from build123d import *

# Parameters (mm, degrees)
F0_W     = 120
F0_H     = 120
F1_DEPTH = 60
F2_W     = 100
F2_H     = 100
F3_DEPTH = 50
F4_R     = 10
F5_R     = 9
F6_DEPTH = 5
F7_R     = 10
F9_DEPTH = 45


with BuildPart() as f1:
    # F0 (on Top) → F1 (new body)
    with BuildSketch(Plane.XY):
        with Locations((-63.325952, -55.072633)):
            Rectangle(F0_W, F0_H)
    extrude(amount=F1_DEPTH)

    # F2 (on face) → F3 (cut)
    with BuildSketch(Plane.XY.offset(60)):
        with Locations((-53.325952, -65.072633)):
            Rectangle(F2_W, F2_H)
    extrude(amount=-F3_DEPTH, mode=Mode.SUBTRACT)

    # F4
    f4_edges = [f1.edges().sort_by_distance(p)[0] for p in [
        (-103.325952, -15.072633, 35),
        (-53.325952, -15.072633, 10),
        (-103.325952, -65.072633, 10),
    ]]
    fillet(f4_edges, radius=F4_R)

    # F5 (on face) → F6 (cut)
    with BuildSketch(Plane.XY.offset(60)):
        with Locations((-63.533046, -10.001782)):
            Circle(F5_R)
    extrude(amount=-F6_DEPTH, mode=Mode.SUBTRACT)

    # F7
    f7_edges = [f1.edges().sort_by_distance(p)[0] for p in [
        (-123.325952, 4.927367, 30),
    ]]
    fillet(f7_edges, radius=F7_R)

    # F8 (on face) → F9 (join)
    with BuildSketch(Plane.XY.offset(10)):
        with BuildLine():
            ThreePointArc((-63.325952, -1.072633), (-72.325952, -10.072633), (-63.325952, -19.072633))
            Line((-63.325952, -19.072633), (-63.325952, -1.072633))
        make_face()
        with BuildLine():
            Line((-63.325952, -1.072633), (-63.325952, -19.072633))
            ThreePointArc((-63.325952, -19.072633), (-56.96199, -16.436594), (-54.325952, -10.072633))
            ThreePointArc((-54.325952, -10.072633), (-56.96199, -3.708672), (-63.325952, -1.072633))
        make_face()
    extrude(amount=F9_DEPTH)


solid = f1.part
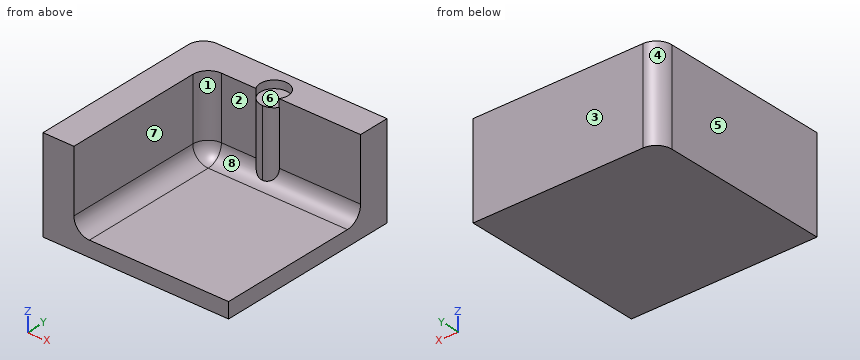
Here's how the part is built. I have some questions about the finished solid (model axes, mm). Face numbers are marked on the shaded views. A direction names the side the tool comes from. Give positions to 0.01 mm unless a question says otherwise; leave off trailing zeros. Order: outer loops, then holes, each group sorted by start corner. A loop starts at its lowest first (then second) coordinate and runs counter-clockwise, first axis right, second up. Notation, with made-up numbers: (46.25, -15.5) -> (60.25, -15.5) arc R18 ccw to (60.25, 2.5) -> close; hole circle Ø9 at (56, -2.5). An arc over 180 degrees is marked (long way). Use a Markdown table: item, result. Add a question column.
Item 1: Imagine slicing it at A-A on x = -19.5. Please give me the cut outline in (y, z).
Item 2: Imagine slicing it at D-D on z = 17. Please give me the cut outline in (x, y), plus the area to 3 significant figures.
Item 3: Imagine slicing it at C-C on z = 25. Please give me the cut outline in (x, y), plus the area to 3 significant figures.
Item 4: I need wall thicknesses on line 1 (Z direction, x = -87, y = -65); line 2 (X direction, y = -56.5, z = 32); line 3 (Y direction, x = -36.5, z = 40). Which ranges of each line are inside material? Lowest first, please.
Item 5: Will these pins go through, and if not, where does the flat tip stop? pin 1 (1 mm diameter, centred on x = -81.5, y = -84.5, fed in from +Z); pin 2 (5 mm diameter, centred on y = -71.5, z = 19.5, fed in from +X); pin 3 (9 mm diameter, centred on x = -61, y = -9.5, fed in from +Z).
Item 6: If we mould it in two halves opening along X, with no side actions, what happens to the marked faces 1, 2, 3 and 4? For each: pulls with the +X half, pulls with the -X half, needs draft (parallel to the pull), parting line crosses it, or undercut.
Item 7: For the marked faces 5, 6, 7 and 8, which set-ups out of +Z, -Z, +X, -X, +Y, -Y let a thin tool reach every point of the face, with its end or its side?
Item 8: Imagine slicing it at B-B on y = -79.5. Please give me the cut outline in (x, z), plus the area to 3 significant figures.
Data:
| question | item | result |
|---|---|---|
| 1 | outline | (-115.07, 0) -> (4.93, 0) -> (4.93, 60) -> (-15.07, 60) -> (-15.07, 20) arc R10 cw to (-25.07, 10) -> (-115.07, 10) -> close |
| 2 | outline | (-123.33, -115.07) -> (-102.87, -115.07) -> (-102.87, -25.07) arc R9.54 cw to (-93.33, -15.53) -> (-70.48, -15.53) arc R9 ccw to (-63.33, -19.07) arc R9 ccw to (-56.17, -15.53) -> (-3.33, -15.53) -> (-3.33, 4.93) -> (-113.33, 4.93) arc R10 ccw to (-123.33, -5.07) -> close |
| 2 | area | 4,530 mm² |
| 3 | outline | (-123.33, -115.07) -> (-103.33, -115.07) -> (-103.33, -25.07) arc R10 cw to (-93.33, -15.07) -> (-70.81, -15.07) arc R9 ccw to (-63.33, -19.07) arc R9 ccw to (-55.84, -15.07) -> (-3.33, -15.07) -> (-3.33, 4.93) -> (-113.33, 4.93) arc R10 ccw to (-123.33, -5.07) -> close |
| 3 | area | 4,440 mm² |
| 4 | line 1 | z = 0 to 10 |
| 4 | line 2 | x = -123.33 to -103.33 |
| 4 | line 3 | y = -15.07 to 4.93 |
| 5 | pin 1 | stops at z = 10 |
| 5 | pin 2 | stops at x = -102.87 |
| 5 | pin 3 | stops at z = 55 |
| 6 | face 1 | undercut |
| 6 | face 2 | undercut |
| 6 | face 3 | needs draft |
| 6 | face 4 | pulls with the -X half |
| 7 | face 5 | +Z, -Z, -X, +Y, -Y |
| 7 | face 6 | +Z |
| 7 | face 7 | +Z, +X, -Y |
| 7 | face 8 | +Z, -Y |
| 8 | outline | (-123.33, 0) -> (-3.33, 0) -> (-3.33, 10) -> (-93.33, 10) arc R10 cw to (-103.33, 20) -> (-103.33, 60) -> (-123.33, 60) -> close |
| 8 | area | 2,220 mm² |
